The model under review builds one solid part; all positions refer to its coordinate system, in mm. Round coordinates to 2 decimals unless told otherwise and drop trailing zeros. Loops run counter-clockwise (first coordinate to the right, second up) from the corner with the lowest first, then second, coordinate; pieces in that order, holes last. Notation, with made-up numbers: M -27,-24 L -2,-24 A25 ccw -2,-3 Z; hole C 10.25,48 d5. An arc over 180 degrees is marked long. Use a Markdown table: item, result. Add a question column.
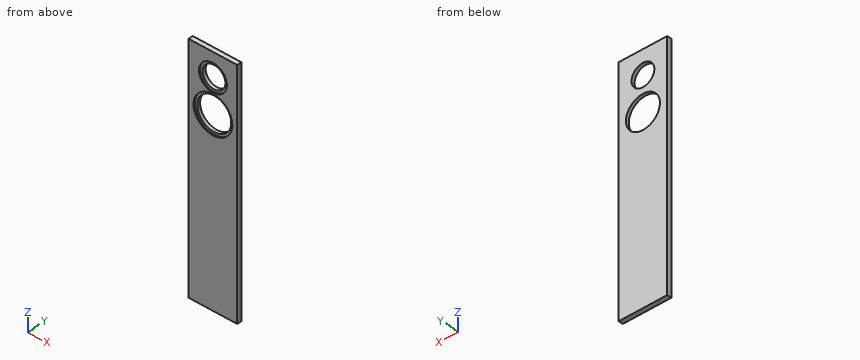
```python
from build123d import *

# Parameters (mm, degrees)
F0_W     = 200
F0_H     = 1000
F1_DEPTH = 19
F2_R     = 57.5
F3_DEPTH = 5
F4_R     = 47
F5_DEPTH = 25
F6_R     = 80
F7_DEPTH = 6
F8_R     = 70
F9_DEPTH = 25


# Not quite as in the source:
# - a feature names something its author has since deleted; it is built from what else it names


with BuildPart() as f1:
    # F0 (on Front) → F1 (new body)
    with BuildSketch(Plane.XZ):
        Rectangle(F0_W, F0_H)
    extrude(amount=F1_DEPTH)

    # F2 (on face) → F3 (cut)
    with BuildSketch(Plane.XZ.offset(19)):
        with Locations((0, 400)):
            Circle(F2_R)
    extrude(amount=-F3_DEPTH, mode=Mode.SUBTRACT)

    # F4 (on face) → F5 (cut)
    with BuildSketch(Plane.XZ.offset(19)):
        with Locations((0, 400)):
            Circle(F4_R)
    extrude(amount=-F5_DEPTH, mode=Mode.SUBTRACT)

    # F6 (on face) → F7 (cut)
    with BuildSketch(Plane.XZ.offset(19)):
        with Locations((0, 257.5)):
            Circle(F6_R)
    extrude(amount=-F7_DEPTH, mode=Mode.SUBTRACT)

    # F8 (on face) + F0 (on Front) → F9 (cut)
    with BuildSketch(Plane.XZ.offset(19)):
        with Locations((0, 257.5)):
            Circle(F8_R)
    with BuildSketch(Plane.XZ):
        Rectangle(F0_W, F0_H)
    extrude(amount=-F9_DEPTH, mode=Mode.SUBTRACT)


solid = f1.part
```
(1) Consider section D-D, the plane x = 25. Give the boundary of the cut face in (y, z), then the cut area to 3 significant figures.
(2) To check wall thickness, follow probe 1 along Z at (x, y) = (0, -7); probe 2 along Z at (x, y) = (0, -17.8); probe 3 along X at (y, z) = (-6.5, 384). State the ranges of each line that lie inside material, in increasing order.
(3) Consider section A-A, the plane z = 257.5. Give the boundary of the cut face in (x, y).
(4) Consider section B-B, the plane x = -27. Give the boundary of the cut face in (y, z).
(5) Consider section C-C, the plane y = -5.25. Give the boundary of the cut face in (x, z).
Found:
| question | item | result |
|---|---|---|
| 1 | outline | M -19,-500 L 0,-500 L 0,192.12 L -13,192.12 L -13,181.51 L -19,181.51 Z; M -19,333.49 L -13,333.49 L -13,322.88 L 0,322.88 L 0,360.2 L -14,360.2 L -14,348.22 L -19,348.22 Z; M -19,451.78 L -14,451.78 L -14,439.8 L 0,439.8 L 0,500 L -19,500 Z |
| 1 | area | 14,800 mm^2 |
| 2 | probe 1 | z = -500 to 187.5, 327.5 to 353, 447 to 500 |
| 2 | probe 2 | z = -500 to 177.5, 337.5 to 342.5, 457.5 to 500 |
| 2 | probe 3 | x = -100 to -44.19, 44.19 to 100 |
| 3 | outline | M -100,-19 L -80,-19 L -80,-13 L -70,-13 L -70,0 L -100,0 Z; M 70,-13 L 80,-13 L 80,-19 L 100,-19 L 100,0 L 70,0 Z |
| 4 | outline | M -19,-500 L 0,-500 L 0,192.92 L -13,192.92 L -13,182.19 L -19,182.19 Z; M -19,332.81 L -13,332.81 L -13,322.08 L 0,322.08 L 0,361.53 L -14,361.53 L -14,349.23 L -19,349.23 Z; M -19,450.77 L -14,450.77 L -14,438.47 L 0,438.47 L 0,500 L -19,500 Z |
| 5 | outline | M -100,-500 L 100,-500 L 100,500 L -100,500 Z; hole C 0,257.5 d140; hole C 0,400 d94 |
